from build123d import *

# Parameters (mm, degrees)
F0_W     = 13
F0_H     = 24
F0_W_2   = 9
F0_H_2   = 20
F1_DEPTH = 10
F0_R     = 0.75
F2_DEPTH = 8
F3_DEPTH = 5


with BuildPart() as f1:
    # F0 (on Top) → F1 (new body)
    with BuildSketch(Plane.XY):
        with Locations((8.4202193944, -4.6071633101)):
            Rectangle(F0_W, F0_H)
        with Locations((8.4202193944, -4.6071633101)):
            Rectangle(F0_W_2, F0_H_2, mode=Mode.SUBTRACT)
    extrude(amount=F1_DEPTH)

    # F0 (on Top) → F2 (join)
    with BuildSketch(Plane.XY):
        with Locations((8.4202193944, -4.6071633101)):
            Rectangle(F0_W, F0_H)
        with Locations((8.4202193944, -4.6071633101)):
            Rectangle(F0_W_2, F0_H_2, mode=Mode.SUBTRACT)
        with Locations((8.4202193944, -4.6071633101)):
            Rectangle(F0_W_2, F0_H_2)
        with Locations((5.4202193944, -13.1071633101)):
            Circle(F0_R, mode=Mode.SUBTRACT)
        with Locations((5.4202193944, -11.0071633101)):
            Circle(F0_R, mode=Mode.SUBTRACT)
        with Locations((7.5202193944, -13.1071633101)):
            Circle(F0_R, mode=Mode.SUBTRACT)
        with Locations((5.4202193944, -8.9071633101)):
            Circle(F0_R, mode=Mode.SUBTRACT)
        with Locations((9.3202193944, -13.1071633101)):
            Circle(F0_R, mode=Mode.SUBTRACT)
        with Locations((11.4202193944, -13.1071633101)):
            Circle(F0_R, mode=Mode.SUBTRACT)
        with Locations((5.4202193944, 3.8928366899)):
            Circle(F0_R, mode=Mode.SUBTRACT)
        with Locations((7.5202193944, 3.8928366899)):
            Circle(F0_R, mode=Mode.SUBTRACT)
        with Locations((9.4202193944, 3.8928366899)):
            Circle(F0_R, mode=Mode.SUBTRACT)
        with Locations((11.4202193944, 1.8928366899)):
            Circle(F0_R, mode=Mode.SUBTRACT)
        with Locations((11.4202193944, 3.8928366899)):
            Circle(F0_R, mode=Mode.SUBTRACT)
    extrude(amount=F2_DEPTH)

    # F0 (on Top) → F3 (join)
    with BuildSketch(Plane.XY):
        with Locations((8.4202193944, -4.6071633101)):
            Rectangle(F0_W, F0_H)
        with Locations((8.4202193944, -4.6071633101)):
            Rectangle(F0_W_2, F0_H_2, mode=Mode.SUBTRACT)
    extrude(amount=-F3_DEPTH)


solid = f1.part
Geometry check sheet. Reference: the model listing, model coordinates, mm. A direction names the side the tool comes from. Coordinates: 2 decimals unless noted, no trailing zeros. Order: outer loops, then holes, each group sorted by start corner. A loop starts at its lowest first (then second) coordinate and runs counter-clockwise, first axis right, second up. Notation, with made-up numbers: (86.25, -13) -> (121.25, -13) arc R19 ccw to (121.25, 6) -> close; hole circle Ø11 at (68.25, 48). An arc over 180 degrees is marked (long way). Use a Markdown table: item, result. Add a question column.
1. Cross-section at D-D (y = -4.5). Enter the section's corners in (x, z).
2. Cross-section at B-B (x = 9). Enter the section's corners in (y, z).
3. Cross-section at C-C (z = -2). Enter the section's corners in (x, y), and give its area (3 significant figures).
4. Mould release check, pull along X, two halves, no side actions. Record for faces 4 (the face through (8, -14.607, -2)), 5 (the face through (14, -4, 10)): pulls with the +X half, pulls with the -X half, needs draft (parallel to the pull), parting line crosses it, or undercut.
5. Go/stop test with flat-tipped pins: pin 1 Ø1.5 at (x, y) = (8, -3) entering from -Z; pin 2 Ø1.2 at (x, y) = (5.42, -11.01) entering from -Z; pin 3 Ø2 at (x, y) = (11.42, 1.89) entering from +Z. Record where each tip stops, or that it passes through.
6. Set-up check for faces 1 (the face through (12.92, -5, 9)), 2 (the face through (5.77, -11.67, 3.94)), 3 (the face through (3.92, -5, -2)): record each of +Z, -Z, +X, -X, +Y, -Y from which the full face is reachable in a straight line by a thin tool's end or side.
7. Material ranges on L1, parallel to Y at x = 11.5, z = 0.25; L2, parallel to Y at x = 5.5, z = 7.75; L3, parallel to X at y = 4, z = -2.75, recorded low to high.
8. Cross-section at A-A (y = 4.25). Enter the section's corners in (x, z).
Filled sheet:
| question | item | result |
|---|---|---|
| 1 | outline | (1.92, -5) -> (3.92, -5) -> (3.92, 0) -> (12.92, 0) -> (12.92, -5) -> (14.92, -5) -> (14.92, 10) -> (12.92, 10) -> (12.92, 8) -> (3.92, 8) -> (3.92, 10) -> (1.92, 10) -> close |
| 2 | outline | (-16.61, -5) -> (-14.61, -5) -> (-14.61, 0) -> (-13.79, 0) -> (-13.79, 8) -> (-14.61, 8) -> (-14.61, 10) -> (-16.61, 10) -> close; (-12.43, 0) -> (3.27, 0) -> (3.27, 8) -> (-12.43, 8) -> close; (4.51, 0) -> (5.39, 0) -> (5.39, -5) -> (7.39, -5) -> (7.39, 10) -> (5.39, 10) -> (5.39, 8) -> (4.51, 8) -> close |
| 3 | outline | (1.92, -16.61) -> (14.92, -16.61) -> (14.92, 7.39) -> (1.92, 7.39) -> close; hole (3.92, -14.61) -> (12.92, -14.61) -> (12.92, 5.39) -> (3.92, 5.39) -> close |
| 3 | area | 132 mm2 |
| 4 | face 4 | undercut |
| 4 | face 5 | needs draft |
| 5 | pin 1 | z = 0 |
| 5 | pin 2 | through |
| 5 | pin 3 | z = 8 |
| 6 | face 1 | +Z |
| 6 | face 2 | +Z, -Z |
| 6 | face 3 | -Z |
| 7 | L1 | -16.61 to -13.85, -12.36 to 1.15, 2.64 to 3.15, 4.64 to 7.39 |
| 7 | L2 | -16.61 to -13.85, -12.36 to -11.75, -10.26 to -9.65, -8.16 to 3.15, 4.64 to 7.39 |
| 7 | L3 | 1.92 to 3.92, 12.92 to 14.92 |
| 8 | outline | (1.92, -5) -> (3.92, -5) -> (3.92, 0) -> (4.76, 0) -> (4.76, 8) -> (3.92, 8) -> (3.92, 10) -> (1.92, 10) -> close; (6.08, 0) -> (6.86, 0) -> (6.86, 8) -> (6.08, 8) -> close; (8.18, 0) -> (8.76, 0) -> (8.76, 8) -> (8.18, 8) -> close; (10.08, 0) -> (10.76, 0) -> (10.76, 8) -> (10.08, 8) -> close; (12.08, 0) -> (12.92, 0) -> (12.92, -5) -> (14.92, -5) -> (14.92, 10) -> (12.92, 10) -> (12.92, 8) -> (12.08, 8) -> close |
